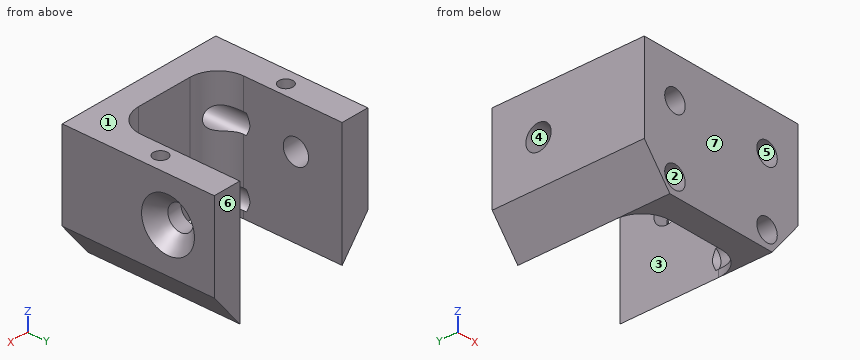
```python
from build123d import *

# Parameters (mm, degrees)
BOSS_EXTRUDE1_DEPTH                                 = 27
SKETCH2_W                                           = 20
SKETCH2_H                                           = 22.5
CUT_EXTRUDE1_DEPTH                                  = 22
BOSS_EXTRUDE2_DEPTH                                 = 22
CSK_FOR_M4_COUNTERSUNK_FLAT_HEAD_SCREW1_D           = 4.5
CSK_FOR_M4_COUNTERSUNK_FLAT_HEAD_SCREW1_DEPTH       = 35
CSK_FOR_M4_COUNTERSUNK_FLAT_HEAD_SCREW1_CSINK_D     = 9.4
CSK_FOR_M4_COUNTERSUNK_FLAT_HEAD_SCREW1_CSINK_ANGLE = 90
CSK_FOR_M4_COUNTERSUNK_FLAT_HEAD_SCREW1_TIP         = 1.351936393
F_2_5MM_DOWEL_HOLE1_D                               = 2.5
F_2_5MM_DOWEL_HOLE1_DEPTH                           = 10
F_2_5MM_DOWEL_HOLE1_TIP                             = 0.751075774
F_4_0MM_DOWEL_HOLE1_D                               = 4
F_4_0MM_DOWEL_HOLE1_DEPTH                           = 10
F_4_0MM_DOWEL_HOLE1_TIP                             = 1.201721238


with BuildPart() as part:
    # Sketch1 → Boss-Extrude1 (new body)
    with BuildSketch(Plane(origin=(0, 0, 0), x_dir=(1, 0, 0), z_dir=(0, 1, 0))):
        Polygon((0, 0), (0, 15.755002002), (5, 22), (25, 22), (30, 15.755002002), (30, 0), align=None)
    extrude(amount=BOSS_EXTRUDE1_DEPTH)

    # Sketch2 → Cut-Extrude1 (cut)
    with BuildSketch(Plane.XY):
        with Locations((15, 15.75)):
            Rectangle(SKETCH2_W, SKETCH2_H)
    extrude(amount=-CUT_EXTRUDE1_DEPTH, mode=Mode.SUBTRACT)

    # Sketch3 → Boss-Extrude2 (add)
    with BuildSketch(Plane.XY):
        with BuildLine():
            Line((5, 9.5), (5, 4.5))
            Line((5, 4.5), (10, 4.5))
            ThreePointArc((10, 4.5), (6.464466094, 5.964466094), (5, 9.5))
        make_face()
        with BuildLine():
            Line((25, 9.5), (25, 4.5))
            Line((25, 4.5), (20, 4.5))
            ThreePointArc((20, 4.5), (23.535533906, 5.964466094), (25, 9.5))
        make_face()
    extrude(amount=-BOSS_EXTRUDE2_DEPTH)

    # CSK for M4 Countersunk Flat Head Screw1
    with Locations(Plane(origin=(30, 0, 0), x_dir=(0, 0, -1), z_dir=(1, 0, 0))):
        with Locations((7.877501001, 18.78691821)):
            CounterSinkHole(CSK_FOR_M4_COUNTERSUNK_FLAT_HEAD_SCREW1_D / 2, CSK_FOR_M4_COUNTERSUNK_FLAT_HEAD_SCREW1_CSINK_D / 2, depth=CSK_FOR_M4_COUNTERSUNK_FLAT_HEAD_SCREW1_DEPTH, counter_sink_angle=CSK_FOR_M4_COUNTERSUNK_FLAT_HEAD_SCREW1_CSINK_ANGLE)
            with Locations((0, 0, -(CSK_FOR_M4_COUNTERSUNK_FLAT_HEAD_SCREW1_DEPTH + CSK_FOR_M4_COUNTERSUNK_FLAT_HEAD_SCREW1_TIP / 2))):  # 118° drill point
                Cone(0, CSK_FOR_M4_COUNTERSUNK_FLAT_HEAD_SCREW1_D / 2, CSK_FOR_M4_COUNTERSUNK_FLAT_HEAD_SCREW1_TIP, mode=Mode.SUBTRACT)

    # Ø2.5mm Dowel Hole1
    with Locations(Plane.XY):
        with Locations((2.75, 14.95), (27.25, 14.95)):
            Hole(F_2_5MM_DOWEL_HOLE1_D / 2, depth=F_2_5MM_DOWEL_HOLE1_DEPTH)
            with Locations((0, 0, -(F_2_5MM_DOWEL_HOLE1_DEPTH + F_2_5MM_DOWEL_HOLE1_TIP / 2))):  # 118° drill point
                Cone(0, F_2_5MM_DOWEL_HOLE1_D / 2, F_2_5MM_DOWEL_HOLE1_TIP, mode=Mode.SUBTRACT)

    # Ø4.0mm Dowel Hole1
    with Locations(Plane(origin=(0, 0, 0), x_dir=(-1, 0, 0), z_dir=(0, -1, 0))):
        with Locations((-24, 19), (-6, 19), (-6, 7.25), (-24, 7.25)):
            Hole(F_4_0MM_DOWEL_HOLE1_D / 2, depth=F_4_0MM_DOWEL_HOLE1_DEPTH)
            with Locations((0, 0, -(F_4_0MM_DOWEL_HOLE1_DEPTH + F_4_0MM_DOWEL_HOLE1_TIP / 2))):  # 118° drill point
                Cone(0, F_4_0MM_DOWEL_HOLE1_D / 2, F_4_0MM_DOWEL_HOLE1_TIP, mode=Mode.SUBTRACT)


solid = part.part
```
Part model, mm, in its own coordinate system. Face numbers are marked on the shaded views. A direction names the side the tool comes from. Give positions to 0.01 mm unless a question says otherwise; leave off trailing zeros. Order: outer loops, then holes, each group sorted by start corner. A loop starts at its lowest first (then second) coordinate and runs counter-clockwise, first axis right, second up. Notation, with made-up numbers: M -30.75,61.25 L -8.75,61.25 A18 ccw -8.75,95.25 Z; hole C -21,27.25 d8. An arc over 180 degrees is marked long. Use a Markdown table: item, result. Add a question column.
(1) Probe line 1 along Z through (x, y) = (24, 3.75); line 2 along X through (y, z) = (25, -7.75); line 3 along Y through (x, z) = (27, -6). List the from-to ranges inside material, lowest first. Write a range as [from, to].
(2) Mould opens along Y. For the marked faces 4, 5, 6 and 7 say: +Y half, -Y half, draft (parallel to the pull), parting line (faces both ways), or undercut.
(3) Saw through at D-D, the plane z = -19. Give the cut face in (x, y), and give its area (3 significant figures).
(4) Saw through at C-C, the plane y = 3.5. Give the cut face in (x, z) (3 decimals), and give its area (3 significant figures).
(5) 3-axis set-ups, long thin cutter, end or side, ignore diameter. For the marked faces 1, 2 and 3: which of +Z, -Z, +X, -X, +Y, -Y reach the whole face in a straight line?
(6) Saw through at A-A, the plane y = 11.5. Give the cut face in (x, z) (3 decimals).
(7) Drop flat-ended pins along their axis: P1, Ø1.5, axis at x = 2.75, y = 14.95, coming from the -Z side; P2, Ø1.5, axis at x = 27.25, y = 14.95, coming from the +Z side; P3, Ø3.5, axis at x = 24, z = -7.25, coming from the -Y side. Give the stop position or say it passes through.
(8) Saw through at B-B, the plane x = 6. Give the cut face in (y, z).
Answer key:
| question | item | result |
|---|---|---|
| 1 | line 1 | [-22, -21], [-17, -9.25], [-5.25, 0] |
| 1 | line 2 | [0, 5], [25, 30] |
| 1 | line 3 | [0, 13.73], [16.17, 17.55], [20.03, 27] |
| 2 | face 4 | undercut |
| 2 | face 5 | draft |
| 2 | face 6 | +Y half |
| 2 | face 7 | -Y half |
| 3 | outline | M 2.6,0 L 4,0 L 4,10 L 5,10.6 L 5,27 L 2.6,27 Z; M 8,0 L 22,0 L 22,4.92 A5 cw 20,4.5 L 10,4.5 A5 cw 8,4.92 Z; M 25,10.6 L 26,10 L 26,0 L 27.4,0 L 27.4,27 L 25,27 Z |
| 3 | area | 173 mm^2 |
| 4 | outline | M 0,-15.755 L 5,-22 L 25,-22 L 30,-15.755 L 30,0 L 0,0 Z; hole C 6,-19 d4; hole C 6,-7.25 d4; hole C 24,-19 d4; hole C 24,-7.25 d4 |
| 4 | area | 579 mm^2 |
| 5 | face 1 | +Z, +X, -X, +Y, -Y |
| 5 | face 2 | -Y |
| 5 | face 3 | +Z, -Z, +Y |
| 6 | outline | M 0,-15.755 L 5,-22 L 5,0 L 0,0 Z; M 25,-22 L 30,-15.755 L 30,0 L 25,0 Z |
| 7 | P1 | z = -20.13 |
| 7 | P2 | z = -10.3 |
| 7 | P3 | y = 10.15 |
| 8 | outline | M 0,-22 L 6.5,-22 L 6.5,-21 L 0,-21 Z; M 0,-17 L 6.5,-17 L 6.5,-9.25 L 0,-9.25 Z; M 0,-5.25 L 6.5,-5.25 L 6.5,0 L 0,0 Z |
